```python
from build123d import *

# Parameters (mm, degrees)
SKETCH_1_R           = 41
SKETCH_1_R_2         = 22.5
EXTRUDE_1_DEPTH      = 40
SKETCH_2_W           = 46
SKETCH_2_H           = 24
EXTRUDE_2_DEPTH      = 10
EXTRUDE_3_REACH      = 249.714
EXTRUDE_3_END_RADIUS = 41
SKETCH_3_W           = 46
SKETCH_3_H           = 18
SKETCH_4_W           = 40.100646326
SKETCH_4_H           = 8
CUT_EXTRUDE_1_DEPTH  = 218.671771252
SKETCH_5_W           = 34
SKETCH_5_H           = 10
CUT_EXTRUDE_2_DEPTH  = 10
FILLET_1_R           = 3
CHAMFER_1_SIZE       = 2


with BuildPart() as part:
    # Sketch 1 → Extrude 1 (new body)
    with BuildSketch(Plane(origin=(0, 0, 0), x_dir=(1, 0, 0), z_dir=(0, 1, 0))):
        with Locations(Location((0, 0, 0), (0, 0, 270))):
            Circle(SKETCH_1_R)
        with Locations(Location((0, 0, 0), (0, 0, 270))):
            Circle(SKETCH_1_R_2, mode=Mode.SUBTRACT)
    extrude(amount=EXTRUDE_1_DEPTH)



with BuildPart() as body_2:
    # Sketch 2 → Extrude 2 (new body)
    with BuildSketch(Plane(origin=(200, 0, 0), x_dir=(0, 0, -1), z_dir=(1, 0, 0))):
        with Locations((0, 20)):
            Rectangle(SKETCH_2_W, SKETCH_2_H)
    extrude(amount=EXTRUDE_2_DEPTH)


with BuildPart() as part_1:
    add(part.part)

    add(body_2.part)  # Extrude 3 merges body 2
    # Extrude 3: up to this cylinder (the profile starts outside it)
    extrude_3_end = Plane(origin=(0, 20, 0), z_dir=(0, -1, 0)) * Cylinder(EXTRUDE_3_END_RADIUS, 582.428, mode=Mode.PRIVATE)
    # Sketch 3 → Extrude 3 (add, up to the surface)
    with BuildSketch(Plane(origin=(200, 0, 0), x_dir=(0, 0, -1), z_dir=(1, 0, 0)), mode=Mode.PRIVATE) as extrude_3_sk1:
        with Locations((0, 20)):
            Rectangle(SKETCH_3_W, SKETCH_3_H)
    extrude_3_tool1 = extrude(extrude_3_sk1.sketch, amount=-EXTRUDE_3_REACH, mode=Mode.PRIVATE) - extrude_3_end
    add(extrude_3_tool1.solids().sort_by_distance((200, 20, 0))[0])

    # Sketch 4 → Cut-Extrude 1 (cut, through all)
    with BuildSketch(Plane(origin=(0, 0, 0), x_dir=(1, 0, 0), z_dir=(0, 1, 0))):
        with Locations((9.949676837, 0)):
            Rectangle(SKETCH_4_W, SKETCH_4_H)
    extrude(amount=CUT_EXTRUDE_1_DEPTH, mode=Mode.SUBTRACT)

    # Sketch 5 → Cut-Extrude 2 (cut, symmetric)
    with BuildSketch(Plane(origin=(200, 0, 0), x_dir=(0, 0, -1), z_dir=(1, 0, 0))):
        with Locations((0, 20)):
            Rectangle(SKETCH_5_W, SKETCH_5_H)
    extrude(amount=CUT_EXTRUDE_2_DEPTH, both=True, mode=Mode.SUBTRACT)

    # Fillet 1
    fillet_1_edges = [part_1.edges().sort_by_distance(p)[0] for p in [
        (116.970562748, 29, 23),
        (116.970562748, 11, 23),
        (116.970562748, 11, -23),
        (116.970562748, 29, -23),
        (0, 0, -41),
        (210, 20, -23),
        (210, 32, 0),
        (210, 20, 23),
        (210, 8, 0),
        (0, 40, -41),
    ]]
    fillet(fillet_1_edges, radius=FILLET_1_R)

    # Chamfer 1
    # the kernel refuses this chamfer: 2.480488228, 2 mm, written as the material it takes off along each edge
    with BuildSketch(Plane(origin=(22.141589825, 47.02037687, 4), x_dir=(1, 0, 0), z_dir=(0, -1, 0))) as chamfer_1_piece_1:
        with BuildLine():
            Line((CHAMFER_1_SIZE, 0), (-0.645316442, 2.645316442))
            ThreePointArc((-0.645316442, 2.645316442), (-0.292721572, 1.373728317), (0, 0))
            Line((0, 0), (CHAMFER_1_SIZE, 0))
        make_face()
    extrude(amount=54.040753739, mode=Mode.SUBTRACT)
    with BuildSketch(Plane(origin=(22.141589825, 47.02037687, -4), x_dir=(1, 0, 0), z_dir=(0, -1, 0))) as chamfer_1_piece_2:
        with BuildLine():
            Line((CHAMFER_1_SIZE, 0), (-0.645316442, -2.645316442))
            ThreePointArc((-0.645316442, -2.645316442), (-0.292721572, -1.373728317), (0, 0))
            Line((0, 0), (CHAMFER_1_SIZE, 0))
        make_face()
    extrude(amount=54.040753739, mode=Mode.SUBTRACT)
    # the kernel refuses this chamfer: 2.480488228, 2 mm, written as the material it takes off along each edge
    with BuildSketch(Plane(origin=(0, 40, 0), x_dir=(0.9975496866331381, 0, 0.06996158015745366), z_dir=(0.06996158015745366, 0, -0.9975496866331381))) as chamfer_1_2_piece_1:
        Polygon((22.5 + CHAMFER_1_SIZE, 0), (22.5, CHAMFER_1_SIZE), (22.5, 0), align=None)
    revolve(axis=Axis((0, 40, 0), (0, -1, 0)), revolution_arc=351.976438974, mode=Mode.SUBTRACT)
    with BuildSketch(Plane(origin=(0, 0, 0), x_dir=(0.9975496866331381, 0, -0.06996158015745378), z_dir=(0.06996158015745378, 0, 0.9975496866331381))) as chamfer_1_2_piece_2:
        Polygon((22.5 + CHAMFER_1_SIZE, 0), (22.5, CHAMFER_1_SIZE), (22.5, 0), align=None)
    revolve(axis=Axis((0, 0, 0), (0, 1, 0)), revolution_arc=351.976438974, mode=Mode.SUBTRACT)


solid = part_1.part
```
Source: CAD feature listing. Evaluate the final solid. Frame: model axes, mm. A direction names the side the tool comes from. Give positions to 0.01 mm unless a question says otherwise; leave off trailing zeros. Order: outer loops, then holes, each group sorted by start corner. A loop starts at its lowest first (then second) coordinate and runs counter-clockwise, first axis right, second up.
(1) Section query B-B (x = 0). Return the cut outline in (y, z), plus the area to 3 significant figures.
(2) Section query C-C (y = 21). Return the cut outline in (x, z).
(3) Material intervals for line 1 along X through (y, z) = (9.5, 11.5); line 2 along X through (y, z) = (31.5, 10.5); line 3 along X through (y, z) = (32.5, -1.5), sorted ascending.
(4) Pull-direction query (Y, two-part tool) for faces 1 (the face through (203, 32, 0)), 2 (the face through (200, 15, 0)), 3 (the face through (-25, 0, -1)); classes: +Y half, -Y half, draft (parallel to the pull), parting line (faces both ways), or undercut.
(5) Section query D-D (x = 171). Return the cut outline in (y, z).
(6) Section query A-A (z = 0). Return the cut outline in (x, y).
(7) Access query for faces 4 (the face through (119, 20, -23)), 5 (the face through (200, 20, -17)), 6 (the face through (27, 20, 4)). Directions: +Z, -Z, +X, -X, +Y, -Y. A direction counts if a zero-diameter tool reaches every point of the face in a straight line with its end or side. Return the directions, or none.
(8) Contact query for flat-ended pins moving along their axis: P1, Ø12, axis at x = 72, y = 27.5, coming from the +Z side; P2, Ø6.5, axis at x = 25.5, y = 21, coming from the +Z side; P3, Ø6.5, axis at x = 27, y = 21, coming from the -Z side; P4, Ø2, axis at x = 181, z = 24.5, coming from the +Y side. Output: stop coordinate, or through.
Outcome:
1. outline: (0, -38) arc R3 ccw to (3, -41) - (37, -41) arc R3 ccw to (40, -38) - (40, -24.5) - (38, -22.5) - (2, -22.5) - (0, -24.5) - close; (0, 24.5) - (2, 22.5) - (38, 22.5) - (40, 24.5) - (40, 38) arc R3 ccw to (37, 41) - (3, 41) arc R3 ccw to (0, 38) - close
1. area: 1,460 mm2
2. outline: (33.94, -23) - (207, -23) arc R3 ccw to (210, -20) - (210, -17) - (190, -17) - (190, 17) - (210, 17) - (210, 20) arc R3 ccw to (207, 23) - (33.94, 23) arc R41 ccw (long way) to start; hole (21.5, -6.65) - (24.14, -4) - (30, -4) - (30, 4) - (24.14, 4) - (21.5, 6.65) arc R22.5 ccw (long way) to start
3. line 1: x = -39.35 to -19.34, 19.34 to 39.35, 200 to 209.6
3. line 2: x = -39.63 to -19.9, 19.9 to 39.63, 200 to 208.66
3. line 3: x = -40.97 to -22.45, 30 to 40.97
4. face 1: +Y half
4. face 2: undercut
4. face 3: -Y half
5. outline: (11, -20) arc R3 ccw to (14, -23) - (26, -23) arc R3 ccw to (29, -20) - (29, 20) arc R3 ccw to (26, 23) - (14, 23) arc R3 ccw to (11, 20) - close
6. outline: (-41, 3) arc R3 ccw to (-38, 0) - (-24.5, 0) - (-22.5, 2) - (-22.5, 38) - (-24.5, 40) - (-38, 40) arc R3 ccw to (-41, 37) - close; (30, 0) - (38, 0) arc R3 ccw to (41, 3) - (41, 11) - (200, 11) - (200, 8) - (207, 8) arc R3 ccw to (210, 11) - (210, 15) - (190, 15) - (190, 25) - (210, 25) - (210, 29) arc R3 ccw to (207, 32) - (200, 32) - (200, 29) - (41, 29) - (41, 37) arc R3 ccw to (38, 40) - (30, 40) - close
7. face 4: -Z, +X, +Y, -Y
7. face 5: +X
7. face 6: +Y, -Y
8. P1: stops at z = 23
8. P2: stops at z = 34.44
8. P3: stops at z = -33.42
8. P4: passes through
